For this review, take the finished solid that the model builds, in its own axes (mm). A direction names the side the tool comes from. Give positions to 0.01 mm unless a question says otherwise; leave off trailing zeros. Order: outer loops, then holes, each group sorted by start corner. A loop starts at its lowest first (then second) coordinate and runs counter-clockwise, first axis right, second up. Notation, with made-up numbers: (57, 64) - (101, 64) arc R23 cw to (101, 77) - close; hole circle Ø7 at (-30, 46.25). An arc over 180 degrees is marked (long way). Use a Markdown table: item, result. Add a question column.
1) Machinability: for faces 5 (the face through (-12, -1, 0)), 6 (the face through (12.02, -3.51, 3.28)), 7 (the face through (-25, 12, -8)), 8 (the face through (25, 10, -7)), which of the approach directions +Z, -Z, +X, -X, +Y, -Y give a long, thin tool a straight path to every point of the face, cutting with its end or side? Answer none if there is none.
2) We need section B-B on y = 5. Write out the cut boundary in (x, z).
3) We need section D-D on z = -2.75. Give the number of separate pieces and of enclosed holes in the cut face, then the cut area to 3 significant figures.
4) Wall thickness on L1, parallel to X at y = -1, z = -4; L2, parallel to Y at x = 14, z = 2.35; L3, parallel to X at y = 2.5, z = -1.75: over which ranges is each line inside the solid? List them lowest first.
5) Clearance check with flat-ended pins moving along their axes: P1, Ø10, axis at x = -24.5, y = 8.5, coming from the -Z side (3 decimals); P2, Ø4, axis at x = 64, y = -1, coming from the -Z side; P3, Ø6.5, axis at x = 13, y = 0.5, coming from the -Z side; P4, Ø2.5, axis at x = -14, y = -1, coming from the +Z side. State where each tip first meets the part, or that it passes through.
6) We need section A-A on x = -64. Write out the cut boundary in (y, z).
7) We need section C-C on x = 37. Write out the cut boundary in (y, z).
8) Mouldability with a two-part tool opening along Y and no side actions: class faces 1 (the face through (-62.57, -0.55, 1.97)), 2 (the face through (0.35, 6.02, -10.46)), 3 (the face through (-47, 0, 0)), 4 (the face through (16, -1, 0)) as released by +Y, released by -Y, zero draft, split by the parting line, or undercut.
```python
from build123d import *

# Parameters (mm, degrees)
SALIENTE_EXTRUIR1_DEPTH    = 4
CROQUIS2_R                 = 1.5
CORTAR_EXTRUIR1_DEPTH      = 13
CORTAR_EXTRUIR1_DEPTH_BACK = 4
SALIENTE_EXTRUIR5_DEPTH    = 94
CORTAR_EXTRUIR2_DEPTH      = 44
CROQUIS10_R                = 1.55
CORTAR_EXTRUIR3_DEPTH      = 44
CORTAR_EXTRUIR3_DEPTH_BACK = 44
CROQUIS15_R                = 4
CORTAR_EXTRUIR5_DEPTH      = 14
CROQUIS17_R                = 1.5
CORTAR_EXTRUIR6_DEPTH      = 16
CROQUIS19_R                = 1.55
CORTAR_EXTRUIR9_DEPTH      = 18
CORTAR_EXTRUIR9_DEPTH_BACK = 9


with BuildPart() as part:
    # Croquis1 → Saliente-Extruir1 (new body)
    with BuildSketch(Plane.XY):
        with BuildLine():
            Line((-66, -19), (66, -19))
            ThreePointArc((66, -19), (68.121320344, -18.121320344), (69, -16))
            Line((69, -16), (69, 16))
            ThreePointArc((69, 16), (68.121320344, 18.121320344), (66, 19))
            Line((66, 19), (-66, 19))
            ThreePointArc((-66, 19), (-68.121320344, 18.121320344), (-69, 16))
            Line((-69, 16), (-69, -16))
            ThreePointArc((-69, -16), (-68.121320344, -18.121320344), (-66, -19))
        make_face()
    extrude(amount=SALIENTE_EXTRUIR1_DEPTH)

    # Croquis2 → Cortar-Extruir1 (cut, two sides)
    with BuildSketch(Plane.XY) as cortar_extruir1_sk:
        with Locations((-64, -1)):
            Circle(CROQUIS2_R)
        with Locations((64, -1)):
            Circle(CROQUIS2_R)
    extrude(amount=CORTAR_EXTRUIR1_DEPTH, mode=Mode.SUBTRACT)
    extrude(cortar_extruir1_sk.sketch, amount=-CORTAR_EXTRUIR1_DEPTH_BACK, mode=Mode.SUBTRACT)

    # Croquis4 → Saliente-Extruir5 (add)
    with BuildSketch(Plane(origin=(69, 0, 0), x_dir=(0, 0, -1), z_dir=(1, 0, 0))):
        Polygon((0, -19), (21.2115146, 31.745163793), (0, 19), align=None)
    extrude(amount=-SALIENTE_EXTRUIR5_DEPTH)

    # Croquis6 → Cortar-Extruir2 (cut)
    with BuildSketch(Plane(origin=(69, 0, 0), x_dir=(0, 0, -1), z_dir=(1, 0, 0))):
        Polygon((0, -19), (0, 19), (21.2115146, 31.745163793), align=None)
    extrude(amount=-CORTAR_EXTRUIR2_DEPTH, mode=Mode.SUBTRACT)

    # Croquis10 → Cortar-Extruir3 (cut, two sides)
    with BuildSketch(Plane.XY.offset(4)) as cortar_extruir3_sk:
        with Locations((-14, -1)):
            Circle(CROQUIS10_R)
        with Locations((14, -1)):
            Circle(CROQUIS10_R)
    extrude(amount=CORTAR_EXTRUIR3_DEPTH, mode=Mode.SUBTRACT)
    extrude(cortar_extruir3_sk.sketch, amount=-CORTAR_EXTRUIR3_DEPTH_BACK, mode=Mode.SUBTRACT)

    # Croquis15 → Cortar-Extruir5 (cut)
    with BuildSketch(Plane.XY):
        with Locations((14, -1)):
            Circle(CROQUIS15_R)
        with Locations((-14, -1)):
            Circle(CROQUIS15_R)
    extrude(amount=-CORTAR_EXTRUIR5_DEPTH, mode=Mode.SUBTRACT)

    # Croquis17 → Cortar-Extruir6 (cut)
    with BuildSketch(Plane(origin=(0, -2.825996258, -6.760745081), x_dir=(-1, 0, 0), z_dir=(0, -0.385663902, -0.922639342))):
        with Locations((-21.6, 28.969852508)):
            Circle(CROQUIS17_R)
    extrude(amount=-CORTAR_EXTRUIR6_DEPTH, mode=Mode.SUBTRACT)

    # Croquis19 → Cortar-Extruir9 (cut, two sides)
    with BuildSketch(Plane(origin=(0, -2.825996258, -6.760745081), x_dir=(-1, 0, 0), z_dir=(0, -0.385663902, -0.922639342))) as cortar_extruir9_sk:
        with Locations((22, -4.530147492)):
            Circle(CROQUIS19_R)
        with Locations((-12, -4.530147492)):
            Circle(CROQUIS19_R)
    extrude(amount=CORTAR_EXTRUIR9_DEPTH, mode=Mode.SUBTRACT)
    extrude(cortar_extruir9_sk.sketch, amount=-CORTAR_EXTRUIR9_DEPTH_BACK, mode=Mode.SUBTRACT)


solid = part.part
```
Checked values:
| question | item | result |
|---|---|---|
| 1 | face 5 | -Z |
| 1 | face 6 | none |
| 1 | face 7 | -Z, -X, +Y, -Y |
| 1 | face 8 | -Z, +X, +Y, -Y |
| 2 | outline | (-69, 0) - (-25, 0) - (-25, -10.03) - (25, -10.03) - (25, 0) - (69, 0) - (69, 4) - (-69, 4) - close |
| 3 | separate pieces | 1 |
| 3 | enclosed holes | 3 |
| 3 | area | 1,540 mm² |
| 4 | L1 | -25 to -18, -10 to 10, 18 to 25 |
| 4 | L2 | -19 to -2.55, 0.55 to 19 |
| 4 | L3 | -25 to -15.94, -12.06 to 12.06, 15.94 to 25 |
| 5 | P1 | z = -13.585 |
| 5 | P2 | z = 0 |
| 5 | P3 | z = -9.51 |
| 5 | P4 | through |
| 6 | outline | (-19, 0) - (-2.5, 0) - (-2.5, 4) - (-19, 4) - close; (0.5, 0) - (19, 0) - (19, 4) - (0.5, 4) - close |
| 7 | outline | (-19, 0) - (19, 0) - (19, 4) - (-19, 4) - close |
| 8 | face 1 | undercut |
| 8 | face 2 | released by -Y |
| 8 | face 3 | zero draft |
| 8 | face 4 | undercut |
